Check sheet for the modelled part. Datum: model origin and axes. Units: mm. A direction names the side the tool comes from. Round coordinates to 2 decimals unless told otherwise and drop trailing zeros. Loops run counter-clockwise (first coordinate to the right, second up) from the corner with the lowest first, then second, coordinate; pieces in that order, holes last. Notation, with made-up numbers: (28, 88) - (76, 88) arc R31 cw to (76, 117) - close; hole circle Ø11 at (-5.75, 10.5). An arc over 180 degrees is marked (long way). Return JSON: item names as keys, results as strings.
from build123d import *

# Parameters (mm, degrees)
SKETCH2_W           = 6
SKETCH2_H           = 6
BOSS_EXTRUDE1_DEPTH = 3
FILLET7_R           = 2
SKETCH3_R           = 2
BOSS_EXTRUDE2_DEPTH = 42.5
FILLET9_R           = 1
BOSS_EXTRUDE3_START = -9.4
SKETCH4_W           = 6
SKETCH4_H           = 6
BOSS_EXTRUDE3_DEPTH = 3
FILLET10_R          = 1


with BuildPart() as part:
    # Sketch2 → Boss-Extrude1 (new body)
    with BuildSketch(Plane(origin=(0, 0, 0), x_dir=(1, 0, 0), z_dir=(0, 1, 0))):
        Rectangle(SKETCH2_W, SKETCH2_H)
    extrude(amount=BOSS_EXTRUDE1_DEPTH)

    # Fillet7
    fillet7_edges = [part.edges().sort_by_distance(p)[0] for p in [
        (3, 1.5, 3),
        (-3, 1.5, 3),
        (-3, 1.5, -3),
        (3, 1.5, -3),
    ]]
    fillet(fillet7_edges, radius=FILLET7_R)

    # Sketch3 → Boss-Extrude2 (add)
    with BuildSketch(Plane(origin=(0, 3, 0), x_dir=(1, 0, 0), z_dir=(0, 1, 0))):
        Circle(SKETCH3_R)
    extrude(amount=BOSS_EXTRUDE2_DEPTH)

    # Fillet9
    fillet9_edges = [part.edges().sort_by_distance(p)[0] for p in [
        (-2, 45.5, 0),
    ]]
    fillet(fillet9_edges, radius=FILLET9_R)

    # Sketch4 → Boss-Extrude3 (add)
    with BuildSketch(Plane(origin=(0, 45.5, 0), x_dir=(1, 0, 0), z_dir=(0, 1, 0)).offset(BOSS_EXTRUDE3_START)):
        Rectangle(SKETCH4_W, SKETCH4_H)
    extrude(amount=-BOSS_EXTRUDE3_DEPTH)

    # Fillet10
    fillet10_edges = [part.edges().sort_by_distance(p)[0] for p in [
        (-3, 34.6, 3),
        (-3, 34.6, -3),
        (3, 34.6, -3),
        (3, 34.6, 3),
    ]]
    fillet(fillet10_edges, radius=FILLET10_R)


solid = part.part
Q1. Scan lines: probe 1 along Y at (x, z) = (2, -1); probe 2 along X at (y, z) = (17, -1.25); probe 3 along Y at (x, z) = (-1.25, 0.5). Record each from-to range of solid material in increasing order. Write a range as [from, to].
Answer key:
{"probe 1": "y = [0, 3], [33.1, 36.1]", "probe 2": "x = [-1.56, 1.56]", "probe 3": "y = [0, 45.44]"}
Q2. Depth check by flat-ended pin: P1, Ø3, axis at x = -2.5, y = 9, coming from the +Z side; P2, Ø2, axis at x = -1, z = 2, coming from the +Y side. Enter the tip coordinate at first touch or a pass-through.
Answer key:
{"P1": "stops at z = 1.73", "P2": "stops at y = 45.47"}
Q3. Sectioned sample at B-B (y = 28). Enter the section's corners in (x, z).
Answer key:
{"outline": "circle Ø4 at (0, 0)"}
Q4. Tool access check on faces 4 (the face through (0, 40, 2)), 5 (the face through (0, 1, 3)), 6 (the face through (1, 33.1, 2)), 7 (the face through (-2.43, 1.52, -2.4)), 8 (the face through (2.43, 1.52, -2.4)). Record the directions out of +Z, -Z, +X, -X, +Y, -Y that give a thin tool (end or side, any length) a straight path to the whole face; none if there is none.
Answer key:
{"face 4": "+Y", "face 5": "+Z, +X, -X, +Y, -Y", "face 6": "none", "face 7": "-Z, -X, -Y", "face 8": "-Z, +X, -Y"}
Q5. Draft check along Y on faces 1 (the face through (0, 18, 2)), 2 (the face through (-2.715, 34.579, 2.699)), 3 (the face through (1, 36.1, 2)). Enter one of: released by +Y, released by -Y, zero draft, split by the parting line, or undercut.
Answer key:
{"face 1": "undercut", "face 2": "zero draft", "face 3": "released by +Y"}
Q6. Sectioned sample at A-A (z = -2.5). Enter the section's corners in (x, y), plus the area to 3 significant figures.
Answer key:
{"outline": "(-2.87, 33.1) - (2.87, 33.1) - (2.87, 36.1) - (-2.87, 36.1) - close; (-2.32, 0) - (2.32, 0) - (2.32, 3) - (-2.32, 3) - close", "area": "31.1 mm²"}
